Verification items for the finished model (mm, model axes). Face numbers are marked on the shaded views. A direction names the side the tool comes from. Give positions to 0.01 mm unless a question says otherwise; leave off trailing zeros. Loops run counter-clockwise (first coordinate to the right, second up) from the corner with the lowest first, then second, coordinate; pieces in that order, holes last. Notation, with made-up numbers: (55, 60) - (92, 60) arc R21 ccw to (92, 83) - close; hole circle Ø7 at (5.5, -14). An arc over 180 degrees is marked (long way). One line per question, with ' | ' between items. Start each with the question number.
1. Section check C-C, the plane y = -9. Enter the section's corners in (x, z), then the cut area to 3 significant figures.
2. Section check A-A, the plane y = -15. Enter the section's corners in (x, z), then the cut area to 3 significant figures.
3. Thickness scan on line 1 along Z through (x, y) = (3.75, -11); line 2 along X through (y, z) = (-9, 24); line 3 along Y through (x, z) = (0, 23.45). Record the ranges inside material, lowest first. Write a range as from..to.
4. Depth check by flat-ended pin: pin 1 Ø2 at (y, z) = (-3.5, 41.5) entering from +X; pin 2 Ø1 at (x, y) = (-4, -4) entering from +Z; pin 3 Ø4 at (x, y) = (1.5, -11.5) entering from -Z; pin 4 Ø3.5 at (x, z) = (-0.5, 39) entering from -Y. Enter the tip coordinate at first touch or a pass-through.
5. Mould release check, pull along Z, two halves, no side actions. Record for the marked faces 4 and 5: +Z half, -Z half, draft (parallel to the pull), parting line (faces both ways), or undercut.
6. Tool access check on the marked faces 1, 2 and 3. Record the directions out of +Z, -Z, +X, -X, +Y, -Y that give a thin tool (end or side, any length) a straight path to the whole face; none if there is none.
7. Section check B-B, the plane x = 0. Enter the section's corners in (y, z).
8. Section check D-D, the plane z = 45. Enter the section's corners in (x, y).
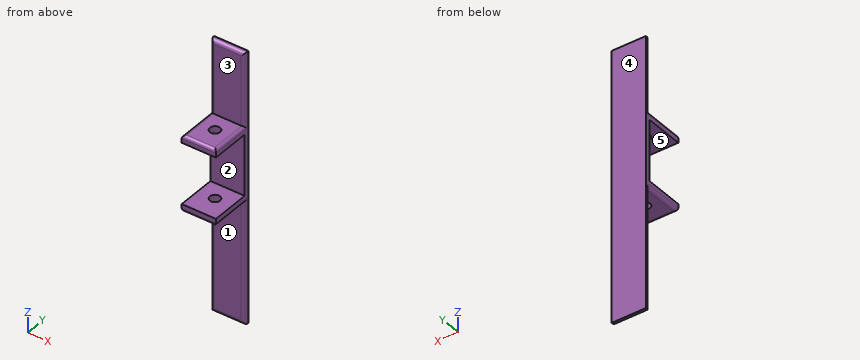
from build123d import *

# Parameters (mm, degrees)
SKETCH_W     = 14
SKETCH_H     = 111
PAD_DEPTH    = 2
SKETCH001_W  = 14
SKETCH001_H  = 3
PAD001_DEPTH = 16
SKETCH002_W  = 14
SKETCH002_H  = 3
PAD002_DEPTH = 16
SKETCH003_R  = 2.1
POCKET_DEPTH = 61.001
FILLET_R     = 1.5
FILLET001_R  = 1.2


with BuildPart() as part:
    # Sketch → Pad (new body)
    with BuildSketch(Plane.XZ):
        Rectangle(SKETCH_W, SKETCH_H)
    extrude(amount=PAD_DEPTH)

    # Sketch001 (on Face6 of Pad) → Pad001 (join)
    with BuildSketch(Plane.XZ.offset(2)):
        with Locations((0, 24)):
            Rectangle(SKETCH001_W, SKETCH001_H)
    extrude(amount=PAD001_DEPTH)

    # Sketch002 (on Face7 of Pad001) → Pad002 (join)
    with BuildSketch(Plane.XZ.offset(2)):
        with Locations((0, -4)):
            Rectangle(SKETCH002_W, SKETCH002_H)
    extrude(amount=PAD002_DEPTH)

    # Sketch003 (on Face14 of Pad002) → Pocket (cut, through all)
    with BuildSketch(Plane(origin=(0, 0, -5.5), x_dir=(1, 0, 0), z_dir=(0, 0, -1))):
        with Locations((0, 9)):
            Circle(SKETCH003_R)
    extrude(amount=-POCKET_DEPTH, mode=Mode.SUBTRACT)

    # Fillet
    fillet_edges = [part.edges().sort_by_distance(p)[0] for p in [
        (7, -2, 40.5),
        (-7, -2, 40.5),
        (0, -2, 55.5),
        (-7, -2, -30.5),
        (7, -2, -30.5),
        (0, -2, -55.5),
    ]]
    fillet(fillet_edges, radius=FILLET_R)

    # Fillet001
    fillet001_edges = [part.edges().sort_by_distance(p)[0] for p in [
        (-7, -10, 25.5),
        (0, -18, 25.5),
        (7, -10, 25.5),
        (0, -18, -5.5),
        (7, -10, -5.5),
        (-7, -10, -5.5),
    ]]
    fillet(fillet001_edges, radius=FILLET001_R)


solid = part.part
Results list:
1) outline: (-7, -4.3) arc R1.2 ccw to (-5.8, -5.5) - (-2.1, -5.5) - (-2.1, -2.5) - (-7, -2.5) - close; (-7, 22.5) - (-2.1, 22.5) - (-2.1, 25.5) - (-5.8, 25.5) arc R1.2 ccw to (-7, 24.3) - close; (2.1, -5.5) - (5.8, -5.5) arc R1.2 ccw to (7, -4.3) - (7, -2.5) - (2.1, -2.5) - close; (2.1, 22.5) - (7, 22.5) - (7, 24.3) arc R1.2 ccw to (5.8, 25.5) - (2.1, 25.5) - close | area: 57.6 mm²
2) outline: (-7, -4.3) arc R1.2 ccw to (-5.8, -5.5) - (5.8, -5.5) arc R1.2 ccw to (7, -4.3) - (7, -2.5) - (-7, -2.5) - close; (-7, 22.5) - (7, 22.5) - (7, 24.3) arc R1.2 ccw to (5.8, 25.5) - (-5.8, 25.5) arc R1.2 ccw to (-7, 24.3) - close | area: 82.8 mm²
3) line 1: -5.5..-2.5, 22.5..25.5 | line 2: -7..-2.1, 2.1..7 | line 3: -18..-11.1, -6.9..0
4) pin 1: through | pin 2: z = 25.5 | pin 3: z = -5.5 | pin 4: y = -2
5) face 4: draft | face 5: undercut
6) face 1: -Z, +X, -X, -Y | face 2: +X, -X, -Y | face 3: +Z, +X, -X, -Y
7) outline: (-18, -4.3) arc R1.2 ccw to (-16.8, -5.5) - (-11.1, -5.5) - (-11.1, -2.5) - (-18, -2.5) - close; (-18, 22.5) - (-11.1, 22.5) - (-11.1, 25.5) - (-16.8, 25.5) arc R1.2 ccw to (-18, 24.3) - close; (-6.9, -5.5) - (-2, -5.5) - (-2, -54) arc R1.5 ccw to (-0.5, -55.5) - (0, -55.5) - (0, 55.5) - (-0.5, 55.5) arc R1.5 ccw to (-2, 54) - (-2, 25.5) - (-6.9, 25.5) - (-6.9, 22.5) - (-2, 22.5) - (-2, -2.5) - (-6.9, -2.5) - close
8) outline: (-7, -0.5) arc R1.5 ccw to (-5.5, -2) - (5.5, -2) arc R1.5 ccw to (7, -0.5) - (7, 0) - (-7, 0) - close
